from build123d import *

# Parameters (mm, degrees)
SKETCH1_W           = 122.771416508
SKETCH1_H           = 67.364835681
BOSS_EXTRUDE1_DEPTH = 50
SKETCH2_W           = 116.771416508
SKETCH2_H           = 61.364835681
CUT_EXTRUDE1_DEPTH  = 47
SKETCH3_R           = 1.676937057
CUT_EXTRUDE3_DEPTH  = 3
FILLET7_R           = 50
FILLET8_R           = 50
FILLET9_R           = 50
FILLET10_R          = 50
FILLET11_R          = 10
FILLET12_R          = 10


with BuildPart() as part:
    # Sketch1 → Boss-Extrude1 (new body)
    with BuildSketch(Plane(origin=(0, 0, 0), x_dir=(1, 0, 0), z_dir=(0, 1, 0))):
        with Locations((61.385708254, 33.682417841)):
            Rectangle(SKETCH1_W, SKETCH1_H)
    extrude(amount=BOSS_EXTRUDE1_DEPTH)

    # Sketch2 → Cut-Extrude1 (cut)
    with BuildSketch(Plane(origin=(0, 50, 0), x_dir=(1, 0, 0), z_dir=(0, 1, 0))):
        with Locations((61.385708254, 33.682417841)):
            Rectangle(SKETCH2_W, SKETCH2_H)
    extrude(amount=-CUT_EXTRUDE1_DEPTH, mode=Mode.SUBTRACT)

    # Sketch3 → Cut-Extrude3 (cut)
    with BuildSketch(Plane.XY):
        with Locations((46.583182692, 23.569957767)):
            Circle(SKETCH3_R)
        with Locations((64.912755506, 18.942876873)):
            Circle(SKETCH3_R)
        with Locations((82.439773274, 23.569957767)):
            Circle(SKETCH3_R)
    extrude(amount=-CUT_EXTRUDE3_DEPTH, mode=Mode.SUBTRACT)

    # Fillet7
    fillet7_edges = [part.edges().sort_by_distance(p)[0] for p in [
        (119.771416508, 26.5, -64.364835681),
    ]]
    fillet(fillet7_edges, radius=FILLET7_R)

    # Fillet8
    fillet8_edges = [part.edges().sort_by_distance(p)[0] for p in [
        (122.771416508, 25, -67.364835681),
    ]]
    fillet(fillet8_edges, radius=FILLET8_R)

    # Fillet9
    fillet9_edges = [part.edges().sort_by_distance(p)[0] for p in [
        (3, 26.5, -64.364835681),
    ]]
    fillet(fillet9_edges, radius=FILLET9_R)

    # Fillet10
    fillet10_edges = [part.edges().sort_by_distance(p)[0] for p in [
        (0, 25, -67.364835681),
    ]]
    fillet(fillet10_edges, radius=FILLET10_R)

    # Fillet11
    fillet11_edges = [part.edges().sort_by_distance(p)[0] for p in [
        (119.771416508, 3, -8.682417841),
        (61.385708254, 3, -64.364835681),
        (105.126755567, 3, -49.720174741),
        (3, 3, -8.682417841),
        (17.644660941, 3, -49.720174741),
    ]]
    fillet(fillet11_edges, radius=FILLET11_R)

    # Fillet12
    fillet12_edges = [part.edges().sort_by_distance(p)[0] for p in [
        (122.771416508, 0, -8.682417841),
        (61.385708254, 0, -67.364835681),
        (108.126755567, 0, -52.720174741),
        (0, 0, -8.682417841),
        (14.644660941, 0, -52.720174741),
    ]]
    fillet(fillet12_edges, radius=FILLET12_R)


solid = part.part
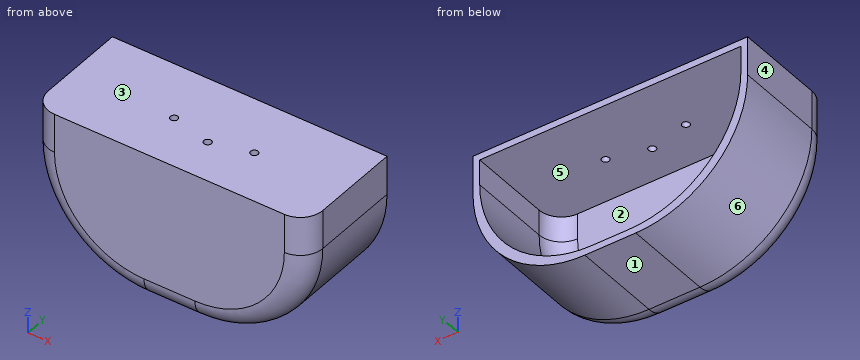
Design review of the part built by this model. Coordinates are the model's own, in mm. Face numbers are marked on the shaded views. A direction names the side the tool comes from. Round coordinates to 2 decimals unless told otherwise and drop trailing zeros. Loops run counter-clockwise (first coordinate to the right, second up) from the corner with the lowest first, then second, coordinate; pieces in that order, holes last. Notation, with made-up numbers: (-9, 68.25) - (48, 68.25) arc R19 cw to (48, 104.25) - close; hole circle Ø4 at (-38.75, 45). An arc over 180 degrees is marked (long way). One line per item, written item: value. Start each with the question number.
1) Consider section C-C on y = 6. Give the boundary of the cut face in (x, z), then the cut area to 3 significant figures.
2) Consider section B-B on x = 55. Give the boundary of the cut face in (y, z), then the cut area to 3 significant figures.
3) Insertion check: pin 1 Ø2 at (x, z) = (44, -55) entering from +Y; pin 2 Ø3 at (x, y) = (26, 44) entering from -Z; pin 3 Ø3 at (x, z) = (60, -51) entering from +Y. Each pin has a flat end and moves straight along its axis. Give the tip position at first contact, or say it passes through.
4) For the marked faces 5 and 6, list the 3-axis set-ups (+Z, -Z, +X, -X, +Y, -Y) from which the entire face can be reached by the end or side of a thin tool; tool diameter is ignored.
5) Draft analysis for pull direction Z (two halves, no side actions). For the marked faces 1, 2, 3 and 4, state which applies: +Z half, -Z half, draft (parallel to the pull), parting line (faces both ways), or undercut.
6) To check wall thickness, follow L1, parallel to Z at x = 52.5, y = 13.5; L2, parallel to Y at x = 94, z = -37; L3, parallel to X at y = 18.5, z = -11.5. State the ranges of each line that lie inside material, in increasing order. Write a range as from..to.
7) Consider section A-A on y = 46. Give the boundary of the cut face in (x, z), then the cut area to 3 significant figures.
Reported:
1. outline: (0.83, -17.36) arc R49.17 ccw to (50, -66.53) - (72.77, -66.53) arc R49.17 ccw to (121.94, -17.36) - (121.94, 0) - (0.83, 0) - close; hole (5.86, -14.36) arc R47.14 ccw to (53, -61.51) - (69.77, -61.51) arc R47.14 ccw to (116.91, -14.36) - (116.91, -3) - (5.86, -3) - close
1. area: 1,480 mm^2
2. outline: (0, -57.36) arc R10 ccw to (10, -67.36) - (50, -67.36) - (50, -64.36) - (13, -64.36) arc R10 cw to (3, -54.36) - (3, -3) - (50, -3) - (50, 0) - (0, 0) - close
2. area: 484 mm^2
3. pin 1: stops at y = 3.35
3. pin 2: stops at z = -62.02
3. pin 3: stops at y = 3
4. face 5: +Y
4. face 6: -Z, -X, +Y, -Y
5. face 1: -Z half
5. face 2: undercut
5. face 3: +Z half
5. face 4: draft
6. L1: z = -67.36..-64.36, -3..0
6. L2: y = 0..3
6. L3: x = 0..3, 119.77..122.77
7. outline: (0, -17.36) arc R50 ccw to (50, -67.36) - (72.77, -67.36) arc R50 ccw to (122.77, -17.36) - (122.77, 0) - (0, 0) - close; hole (3, -14.36) arc R50 ccw to (53, -64.36) - (69.77, -64.36) arc R50 ccw to (119.77, -14.36) - (119.77, -3) - (3, -3) - close
7. area: 1,100 mm^2
